Autodesk Inventor part; units mm, degrees
ref_plane "YZ Plane" through (0, 0, 0) normal (1, 0, 0) x (0, 1, 0)
ref_plane "XZ Plane" through (0, 0, 0) normal (0, 1, 0) x (-1, 0, 0)
ref_plane "XY Plane" through (0, 0, 0) normal (0, 0, 1) x (1, 0, 0)
sketch "Sketch1" plane through (0, 0, 0) normal (0, 0, 1) x (1, 0, 0)
  line L0 (20, 22.75) -> (-20, 22.75)
  line L1 (8, 74.45) -> (-8, 74.45)
  line L2 (0, 22.75) -> (0, 133.134)
  line L3 (28.8904, 63.2) -> (28.8904, 73.2)
  line L4 (28.8904, 73.2) -> (0, 102.0904)
  line L5 (28.8904, 73.2) -> (69.7476, 73.2) construction
  line L6 (0, 102.0904) -> (-36.5211, 65.5693)
  line L7 (0, 102.0904) -> (148.4924, -46.402)
  line L8 (148.4924, -46.402) -> (0, -194.8944)
  line L9 (0, -194.8944) -> (-148.4924, -46.402)
  line L10 (-148.4924, -46.402) -> (0, 102.0904)
  line L11 (0, 102.0904) -> (210, 102.0904) construction
  point P0 (0, 0)
  dimension "d0" = 135
  dimension "d1" = 90
  dimension "d2" = 210
  dimension "d3" = 45
  dimension "d4" = 210
extrude "Extrusion1" add sketch "Sketch1" along normal blind 3.5
sketch "Sketch2" plane through (0, 0, 0) normal (0, 0, -1) x (-1, 0, 0)
  line L0 (0, 102.0904) -> (148.4924, -46.402)
  line L1 (-148.4924, -46.402) -> (0, 102.0904)
  line L2 (0, -194.8944) -> (-148.4924, -46.402)
  line L3 (148.4924, -46.402) -> (0, -194.8944)
  line L4 (-148.4924, -46.402) -> (148.4924, -46.402)
  line L5 (0, -194.8944) -> (0, 102.0904)
  circle A0 centre (0, -46.402) radius 25
  point P0 (0, 0)
  dimension "d8" = 50
extrude "Extrusion2" cut sketch "Sketch2" against normal blind 50 contours A0 L4 L5 | L5 L4 A0 | A0 L5 L4 | L4 L5 A0
equation "\"d9\" = d8"
properties part number "MainBase210"
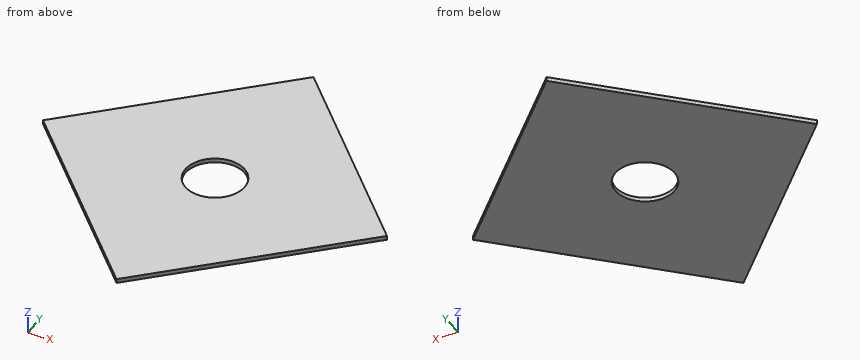
Read the model definition and answer for the solid it produces. Units are mm, in the model's axes. Coordinates: 2 decimals unless noted, no trailing zeros. Loops run counter-clockwise (first coordinate to the right, second up) from the corner with the lowest first, then second, coordinate; pieces in that order, holes last.
Q1. Consider probe 1 along Y at (x, z) = (0, 1.55); probe 2 along X at (y, z) = (-178.5, 2.65); probe 3 along X at (y, z) = (-156, 2.45). Determine where each line is inside the solid, lowest interval first.
Q2. The part is cut by section C-C on y = -84. Write down the section's boundary in (x, z).
Q3. The part is cut by section B-B on x = 127.5. Write down the section's boundary in (y, z).
Q4. Each of these flat-tipped pins is pushed along its axis until it touches: pin 1 Ø1.5 at (x, z) = (16, 2) entering from +Y; pin 2 Ø2 at (y, z) = (-66.5, 1.5) entering from -X; pin 3 Ø1.5 at (y, z) = (-18, 3) entering from +X. Where does it stop, or does it pass through?
Q5. The part is cut by section A-A on y = -38. Write down the section's boundary in (x, z), and give its area (3 significant figures).
Results below:
1. probe 1: y = -194.89 to -71.4, -21.4 to 102.09
1. probe 2: x = -16.39 to 16.39
1. probe 3: x = -38.89 to 38.89
2. outline: (-110.89, 0) - (110.89, 0) - (110.89, 3.5) - (-110.89, 3.5) - close
3. outline: (-67.39, 0) - (-25.41, 0) - (-25.41, 3.5) - (-67.39, 3.5) - close
4. pin 1: stops at y = 86.84
4. pin 2: stops at x = -129.39
4. pin 3: stops at x = 120.84
5. outline: (-140.09, 0) - (-23.55, 0) - (-23.55, 3.5) - (-140.09, 3.5) - close; (23.55, 0) - (140.09, 0) - (140.09, 3.5) - (23.55, 3.5) - close
5. area: 816 mm2
